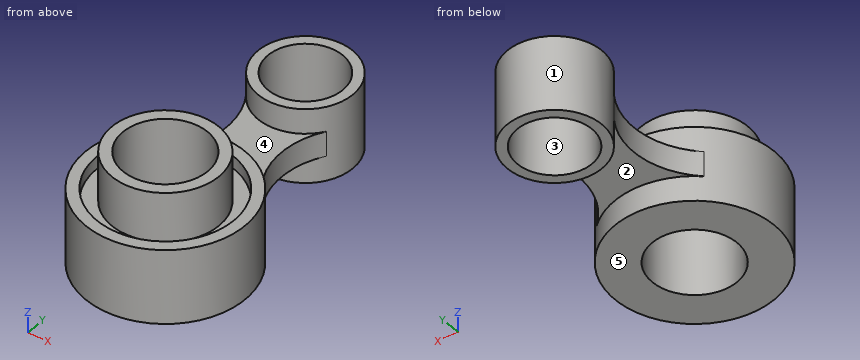
from build123d import *

# Parameters (mm, degrees)
SKETCH1_R           = 32
BOSS_EXTRUDE3_DEPTH = 45
SKETCH4_R           = 17
CUT_EXTRUDE1_DEPTH  = 45
CUT_EXTRUDE2_START  = -15
SKETCH5_R           = 32
SKETCH5_R_2         = 21.5
CUT_EXTRUDE2_DEPTH  = 15
CUT_EXTRUDE3_START  = -5
SKETCH6_R           = 27.5
SKETCH6_R_2         = 21.5
CUT_EXTRUDE3_DEPTH  = 5
SKETCH7_R           = 19
SKETCH7_R_2         = 15
BOSS_EXTRUDE4_DEPTH = 30
BOSS_EXTRUDE5_START = 10
BOSS_EXTRUDE5_DEPTH = 10


with BuildPart() as part:
    # Sketch1 → Boss-Extrude3 (new body)
    with BuildSketch(Plane.XY):
        with Locations(Location((0, 0, 0), (0, 0, 180))):
            Circle(SKETCH1_R)
    extrude(amount=BOSS_EXTRUDE3_DEPTH)

    # Sketch4 → Cut-Extrude1 (cut)
    with BuildSketch(Plane.XY.offset(45)):
        Circle(SKETCH4_R)
    extrude(amount=-CUT_EXTRUDE1_DEPTH, mode=Mode.SUBTRACT)

    # Sketch5 → Cut-Extrude2 (cut)
    with BuildSketch(Plane.XY.offset(45).offset(CUT_EXTRUDE2_START)):
        with Locations(Location((0, 0, 0), (0, 0, 180))):
            Circle(SKETCH5_R)
        Circle(SKETCH5_R_2, mode=Mode.SUBTRACT)
    extrude(amount=CUT_EXTRUDE2_DEPTH, mode=Mode.SUBTRACT)

    # Sketch6 → Cut-Extrude3 (cut)
    with BuildSketch(Plane.XY.offset(30).offset(CUT_EXTRUDE3_START)):
        Circle(SKETCH6_R)
        Circle(SKETCH6_R_2, mode=Mode.SUBTRACT)
    extrude(amount=CUT_EXTRUDE3_DEPTH, mode=Mode.SUBTRACT)



with BuildPart() as body_2:
    # Sketch7 → Boss-Extrude4 (new body)
    with BuildSketch(Plane.XY):
        with Locations((0, 75)):
            Circle(SKETCH7_R)
        with Locations((0, 75)):
            Circle(SKETCH7_R_2, mode=Mode.SUBTRACT)
    extrude(amount=BOSS_EXTRUDE4_DEPTH)


with BuildPart() as part_1:
    add(part.part)

    add(body_2.part)  # Boss-Extrude5 merges body 2
    # Sketch8 → Boss-Extrude5 (add)
    with BuildSketch(Plane.XY.offset(BOSS_EXTRUDE5_START)):
        with BuildLine():
            ThreePointArc((15.993228521, 64.74248366), (11.210252348, 43.234782297), (21.464596173, 23.733333333))
            ThreePointArc((21.464596173, 23.733333333), (0, 32), (-21.464596173, 23.733333333))
            ThreePointArc((-21.464596173, 23.733333333), (-11.210252348, 43.234782297), (-15.993228521, 64.74248366))
            ThreePointArc((-15.993228521, 64.74248366), (0, 56), (15.993228521, 64.74248366))
        make_face()
    extrude(amount=BOSS_EXTRUDE5_DEPTH)


solid = part_1.part
Part model, mm, in its own coordinate system. Face numbers are marked on the shaded views. A direction names the side the tool comes from. Coordinates: 2 decimals unless noted, no trailing zeros. Order: outer loops, then holes, each group sorted by start corner. A loop starts at its lowest first (then second) coordinate and runs counter-clockwise, first axis right, second up. Notation, with made-up numbers: M 53.5,37.5 L 78.5,37.5 A10 ccw 78.5,53.5 Z; hole C -3.75,12 d6. An arc over 180 degrees is marked long. One line per question, with ' | ' between items.
Q1. 3-axis set-ups, long thin cutter, end or side, ignore diameter. For the marked faces 4 and 5: which of +Z, -Z, +X, -X, +Y, -Y reach the whole face in a straight line?
A:
face 4: +Z | face 5: -Z, +X, -X, +Y, -Y
Q2. Slice it at D-D (y = 75). Give the cut face in (x, z), and give its area (3 significant figures).
A:
outline: M -19,0 L -15,0 L -15,30 L -19,30 Z; M 15,0 L 19,0 L 19,30 L 15,30 Z | area: 240 mm^2
Q3. Drill centre lines: line 1 (Y direction, x = 0, z = 26); line 2 (Z direction, x = -8, y = 23); line 3 (Z direction, x = 11, y = 64.5). Where is each one in solid material? Low to high.
A:
line 1: y = -32 to -27.5, -21.5 to -17, 17 to 21.5, 27.5 to 32, 56 to 60, 90 to 94 | line 2: z = 0 to 25 | line 3: z = 0 to 30
Q4. Slice it at C-C (z = 42.5). Give the cut face in (x, y).
A:
outline: C 0,0 d43; hole C 0,0 d34
Q5. Slice it at A-A (x = 0). Give the cut face in (y, z).
A:
outline: M -32,0 L -17,0 L -17,45 L -21.5,45 L -21.5,25 L -27.5,25 L -27.5,30 L -32,30 Z; M 17,0 L 32,0 L 32,10 L 56,10 L 56,0 L 60,0 L 60,30 L 56,30 L 56,20 L 32,20 L 32,30 L 27.5,30 L 27.5,25 L 21.5,25 L 21.5,45 L 17,45 Z; M 90,0 L 94,0 L 94,30 L 90,30 Z
Q6. Two-plate mould, pull along X, no slides. Class the marked faces 1, 2 and 3: +X half, -X half, draft (parallel to the pull), parting line (faces both ways), or undercut.
A:
face 1: parting line | face 2: draft | face 3: undercut
Q7. Slice it at B-B (y = 0). Give the cut face in (x, z), and give its area (3 significant figures).
A:
outline: M -32,0 L -17,0 L -17,45 L -21.5,45 L -21.5,25 L -27.5,25 L -27.5,30 L -32,30 Z; M 17,0 L 32,0 L 32,30 L 27.5,30 L 27.5,25 L 21.5,25 L 21.5,45 L 17,45 Z | area: 975 mm^2
Q8. Pin check, flat tips, straight feed: P1, Ø10, axis at y = 23.5, z = 16.5, coming from the -X side; P2, Ø2, axis at x = 23.5, y = -2.5, coming from the +Z side; P3, Ø4, axis at x = 1.5, y = 60.5, coming from the -Z side; P4, Ø20.5, axis at x = 0, y = 0, coming from the -Z side. Stop position of each tip, or through.
A:
P1: stops at x = -26.11 | P2: stops at z = 25 | P3: stops at z = 0 | P4: passes through
